Source: CAD feature listing. Evaluate the final solid. Frame: model axes, mm. A direction names the side the tool comes from. Give positions to 0.01 mm unless a question says otherwise; leave off trailing zeros. Loops run counter-clockwise (first coordinate to the right, second up) from the corner with the lowest first, then second, coordinate; pieces in that order, holes last. Notation, with made-up numbers: (-26, 0) - (3, 0) arc R26 cw to (3, 28) - close; hole circle Ø7 at (40.25, -34.75). An arc over 180 degrees is marked (long way). Write each question's results on one line, items separated by ' | '. Start each with the question number.
(1) Cut plane B-B on y = 0. Return the cut outline in (x, z).
(2) Cut plane D-D on y = -71. Return the cut outline in (x, z).
(3) Material intervals for line 1 along Y through (x, z) = (0, -7); line 2 along X through (y, z) = (-56, -5.75); line 3 along X through (y, z) = (-6, -2.75), sorted ascending. Write a range as [from, to].
(4) Cut plane C-C on x = 0. Return the cut outline in (y, z).
(5) Cut plane A-A on z = 0. Return the cut outline in (x, y).
(6) Reachability of faces 4 (the flat face through (8, -72, -9)), 5 (the flat face through (9, -72, 8)), 6 (the flat face through (-8, -72, 9)), 7 (the flat face through (12, -41, 0)), 8 (the cylindrical face through (-2.17, -89.86, 9.76)) from +Z, -Z, +X, -X, +Y, -Y: full face, straight path, thin tool, end or side. Return the list, or none.
(7) Pull-direction query (X, two-part tool) for faces 1 (the cylindrical face through (-2.17, 9.76, -0.17)), 2 (the flat face through (0, -29, -12)), 3 (the flat face through (-12, -41, 0)); classes: pulls with the +X half, pulls with the -X half, needs draft (parallel to the pull), parting line crosses it, or undercut.
(8) Contact query for flat-ended pins moving along their axis: pin 1 (4 mm diameter, centred on x = -1, z = -4, fed in from +Y); pin 2 (1.1 mm diameter, centred on x = -11, z = 11, fed in from -Y); pin 3 (0.7 mm diameter, centred on x = -11.5, z = -11, fed in from -Y). Output: stop coordinate, or through.
Solid Edge part; units mm, degrees
sketch "Sketch1" plane through (0, 0, 0) normal (0, 0, 1) x (1, 0, 0)
  circle A0 centre (0, 0) radius 10
  circle A1 centre (0, 0) radius 20
extrude "Protrusion1" add sketch "Sketch1" along normal mid plane 24
sketch "Sketch2" plane through (0, -80, 0) normal (0, -1, 0) x (1, 0, 0)
  line L0 (-12, 12) -> (12, 12)
  line L1 (12, 12) -> (12, -12)
  line L2 (12, -12) -> (-12, -12)
  line L3 (-12, -12) -> (-12, 12)
  dimension "D1" = 12
  dimension "D2" = 12
extrude "Protrusion2" add sketch "Sketch2" against normal up to next
sketch "Sketch3" plane through (0, -80, 0) normal (0, -1, 0) x (1, 0, 0)
  circle A0 centre (0, 0) radius 10
extrude "ExtrudedProtrusion_3" add sketch "Sketch3" along normal blind 20
sketch "Sketch4" plane through (0, -80, 0) normal (0, -1, 0) x (1, 0, 0)
  line L0 (-5, 12) -> (5, 12)
  line L1 (12, 5) -> (5, 12)
  line L2 (12, -5) -> (12, 5)
  line L3 (5, -12) -> (12, -5)
  line L4 (-5, -12) -> (5, -12)
  line L5 (-12, -5) -> (-5, -12)
  line L6 (-12, -5) -> (-12, 5)
  line L7 (-5, 12) -> (-12, 5)
extrude "ExtrudedCutout_1" cut sketch "Sketch4" against normal blind 20 flip side to cut
fillet "Round_1" radius 4 4 edges at (-8.5, -60, 8.5) (8.5, -60, 8.5) (-8.5, -60, -8.5) (8.5, -60, -8.5)
properties part number "2"
Ans:
1) outline: (-20, -12) - (-10, -12) - (-10, 12) - (-20, 12) - close; (10, -12) - (20, -12) - (20, 12) - (10, 12) - close
2) outline: (-12, -5) - (-5, -12) - (5, -12) - (12, -5) - (12, 5) - (5, 12) - (-5, 12) - (-12, 5) - close
3) line 1: [-100, -10], [10, 20] | line 2: [-12, 12] | line 3: [-19.08, -8], [8, 19.08]
4) outline: (-100, -10) - (-80, -10) - (-80, -12) - (-10, -12) - (-10, 12) - (-80, 12) - (-80, 10) - (-100, 10) - close; (10, -12) - (20, -12) - (20, 12) - (10, 12) - close
5) outline: (-12, -80) - (-10, -80) - (-10, -100) - (10, -100) - (10, -80) - (12, -80) - (12, -16) arc R20 ccw (long way) to (-12, -16) - close; hole circle Ø20 at (0, 0)
6) face 4: -Z, +X, -Y | face 5: +Z, +X, -Y | face 6: +Z, -X, -Y | face 7: +Z, -Z, +X, -Y | face 8: -Y
7) face 1: undercut | face 2: needs draft | face 3: pulls with the -X half
8) pin 1: y = 20 | pin 2: y = -60.13 | pin 3: y = -60.03
